For this review, use the dimensioned drawing (mm, ordinates from the lowest corner) and the shaded views. A direction names the side the tool comes from. Coordinates: 2 decimals unless noted, no trailing zeros. Write each loop counter-clockwise with the first axis right and the second up, starting at its lowest first coordinate (ties: lowest second). Pieces come first, ordered by that corner, then holes. Notation, with made-up numbers: M 81,53.5 L 98,53.5 A19 cw 98,66.5 Z; hole C -5,45.25 d5. An arc over 180 degrees is marked long. One line per question, with ' | ' between items.
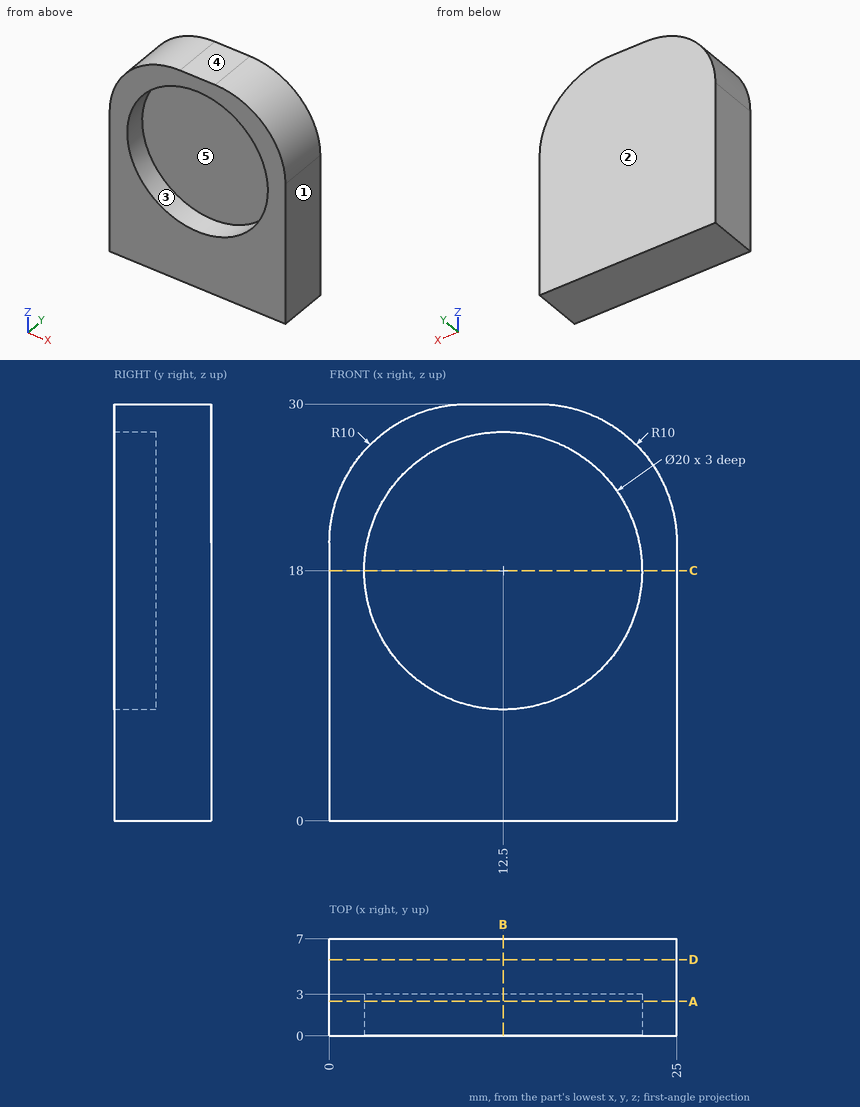
1. Take a section at D-D (y = 5.5). Write out the cut boundary in (x, z).
Answer sheet:
outline: M 0,0 L 25,0 L 25,20 A10 ccw 15,30 L 10,30 A10 ccw 0,20 Z
2. Take a section at C-C (z = 18). Write out the cut boundary in (x, y), then the cut area to 3 significant figures.
Answer sheet:
outline: M 0,0 L 2.5,0 L 2.5,3 L 22.5,3 L 22.5,0 L 25,0 L 25,7 L 0,7 Z | area: 115 mm^2
3. Tool access review of the marked faces 4 and 5: name each direction out of +Z, -Z, +X, -X, +Y, -Y from which nothing blocks a thin tool from reaching the whole face with its end or side.
Answer sheet:
face 4: +Z, +X, -X, +Y, -Y | face 5: -Y
4. Take a section at A-A (y = 2.5). Write out the cut boundary in (x, z).
Answer sheet:
outline: M 0,0 L 25,0 L 25,20 A10 ccw 15,30 L 10,30 A10 ccw 0,20 Z; hole C 12.5,18 d20
5. Take a section at B-B (x = 12.5). Write out the cut boundary in (y, z).
Answer sheet:
outline: M 0,0 L 7,0 L 7,30 L 0,30 L 0,28 L 3,28 L 3,8 L 0,8 Z
6. Draft analysis for pull direction X (two halves, no side actions). For the marked faces 1, 2 and 3, state which applies: pulls with the +X half, pulls with the -X half, needs draft (parallel to the pull), parting line crosses it, or undercut.
Answer sheet:
face 1: pulls with the +X half | face 2: needs draft | face 3: undercut
7. To check wall thickness, follow line 1 along X through (y, z) = (1.05, 18); line 2 along Z through (x, y) = (12.75, 1.5); line 3 along Y through (x, z) = (7.75, 16.25). State the ranges of each line that lie inside material, in increasing order. Write a range as [from, to].
Answer sheet:
line 1: [0, 2.5], [22.5, 25] | line 2: [0, 8], [28, 30] | line 3: [3, 7]
